For this review, use the dimensioned drawing (mm, ordinates from the lowest corner) and the shaded views. Give positions to 0.01 mm unless a question says otherwise; leave off trailing zeros. Loops run counter-clockwise (first coordinate to the right, second up) from the corner with the lowest first, then second, coordinate; pieces in that order, holes last. Notation, with made-up numbers: (63, 53) - (116, 53) arc R23 ccw to (116, 82) - close; hole circle Ø5 at (17.25, 9.25). An arc over 180 degrees is marked (long way). Write each question's results on one line, items separated by ' | '.
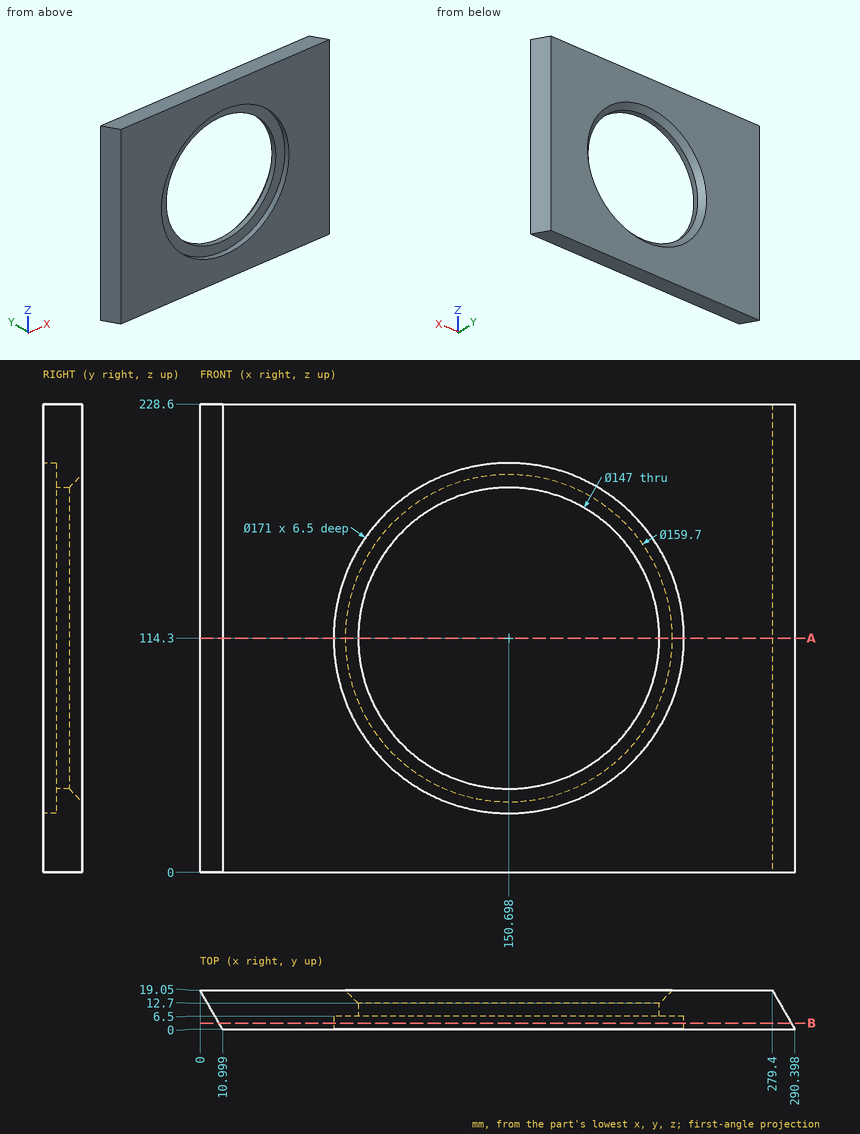
Item 1: Wall thickness on probe 1 along Z at (x, y) = (156, 15.75) (1 decimal); probe 2 along Z at (x, y) = (131, 17.5); probe 3 along Y at (x, z) = (197.5, 44): over which ranges is each line inside the solid? List them lowest first.
Output values:
probe 1: z = 0 to 37.9, 190.7 to 228.6 | probe 2: z = 0 to 38.52, 190.08 to 228.6 | probe 3: y = 6.5 to 19.05
Item 2: Clearance check with flat-ended pins moving along their axes: P1, Ø1.5, axis at y = 6, z = 189, coming from the +X side; P2, Ø1.5, axis at x = 136.5, y = 10, coming from the -Z side; P3, Ø1, axis at y = 5, z = 193.5, coming from the +X side; P4, Ø4, axis at y = 8, z = 49, coming from the +X side (1 decimal). State where each tip first meets the part, or that it passes through.
Output values:
P1: stops at x = 287.37 | P2: stops at z = 0 | P3: stops at x = 287.8 | P4: stops at x = 286.9
Item 3: We need section A-A on z = 114.3. Give the boundary of the cut face in (x, y).
Output values:
outline: (0, 19.05) - (11, 0) - (65.2, 0) - (65.2, 6.5) - (77.2, 6.5) - (77.2, 12.7) - (70.85, 19.05) - close; (224.2, 6.5) - (236.2, 6.5) - (236.2, 0) - (290.4, 0) - (279.4, 19.05) - (230.55, 19.05) - (224.2, 12.7) - close
Item 4: We need section B-B on y = 3. Give the boundary of the cut face in (x, z).
Output values:
outline: (9.27, 0) - (288.67, 0) - (288.67, 228.6) - (9.27, 228.6) - close; hole circle Ø171 at (150.7, 114.3)
